The listing builds one solid part. Answer for the finished solid, in the listing's coordinates (mm). Give positions to 0.01 mm unless a question says otherwise; leave off trailing zeros. Write each loop counter-clockwise with the first axis right and the second up, starting at its lowest first coordinate (ties: lowest second). Pieces come first, ordered by that corner, then holes. Notation, with made-up numbers: (44.25, 37) - (63.25, 37) arc R15 ccw to (63.25, 57) - close; hole circle Ø4 at (-27, -13). An arc over 180 degrees is marked (long way). Use a Markdown table: item, result. Add a question column.
from build123d import *

# Parameters (mm, degrees)
F1_DEPTH = 1.27
F2_SIZE2 = 0.635
F2_SIZE  = 3.81
F3_SIZE2 = 3.80999
F3_SIZE  = 0.63499


# Not quite as in the source:
# - a fillet or chamfer is up to 0.001 mm smaller than in the source, because OpenCascade refuses the exact size


with BuildPart() as f1:
    # F0 (on Top) → F1 (new body)
    with BuildSketch(Plane.XY):
        with BuildLine():
            Line((-36.8330654015, 25.4), (-36.8330654015, 0))
            Line((-36.8330654015, 0), (-31.7530654015, 0))
            Line((-31.7530654015, 0), (-31.7530654015, 25.4))
            Line((-31.7530654015, 25.4), (-31.7530654015, 38.1))
            ThreePointArc((-31.7530654015, 38.1), (-27.5303919686, 58.0516897911), (-36.8330654015, 76.2))
            Line((-36.8330654015, 76.2), (-36.8330654015, 25.4))
        make_face()
    extrude(amount=F1_DEPTH)

    # F2
    f2_edges = [f1.edges().sort_by_distance(p)[0] for p in [
        (-27.530392, 58.05169, 1.27),
    ]]
    f2_side = f1.faces().sort_by_distance((-33.424726, 40.272923, 1.27))[0]
    chamfer(f2_edges, length=F2_SIZE, length2=F2_SIZE2, reference=f2_side)

    # F3 (size 0.635 and 3.81 in the source; OpenCascade refuses exactly that, so slightly less here)
    f3_edges = [f1.edges().sort_by_distance(p)[0] for p in [
        (-27.530392, 58.05169, 0),
    ]]
    f3_side = f1.faces().sort_by_distance((-27.530392, 58.05169, 0.3175))[0]
    chamfer(f3_edges, length=F3_SIZE, length2=F3_SIZE2, reference=f3_side)


solid = f1.part
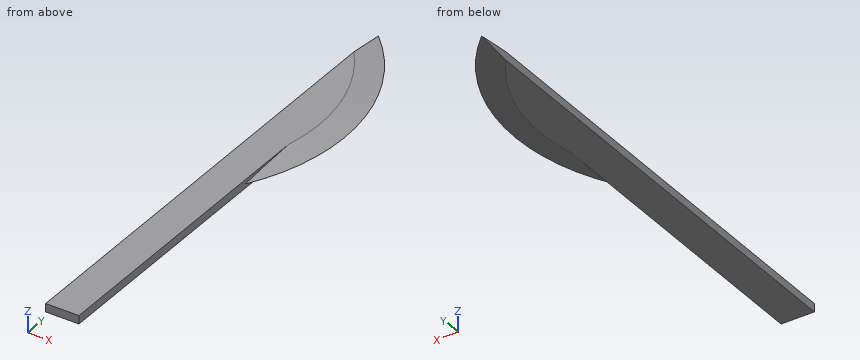
1. Consider L1, parallel to X at y = 7.5, z = 0.45; L2, parallel to Z at x = -28.75, y = 51; L3, parallel to Z at x = -28, y = 56. Determine where each line is inside the solid, lowest interval first. Write a range as [from, to].
2. The part is cut by section A-A (y = 32.5). Give the vertices of the cut face in (x, z), and give its area (3 significant figures).
3. The part is cut by section B-B (z = 0.85). Give the vertices of the cut face in (x, y).
4. Given P1, Ø0.6, axis at y = 32, z = 0.5, coming from the +X side, flat-ended and moving along its own axis, determine where the tip first touches the part or whether it passes through.
Check values:
| question | item | result |
|---|---|---|
| 1 | L1 | x = [-36.83, -31.75] |
| 1 | L2 | z = [0.41, 0.86] |
| 1 | L3 | z = [0.52, 0.75] |
| 2 | outline | (-36.83, 0) - (-31.75, 0) - (-31.75, 1.27) - (-36.83, 1.27) - close |
| 2 | area | 6.45 mm2 |
| 3 | outline | (-36.83, 0) - (-31.75, 0) - (-31.75, 40.74) arc R29.19 ccw to (-36.83, 74.39) - close |
| 4 | P1 | stops at x = -31.75 |
